Part model, mm, in its own coordinate system. A direction names the side the tool comes from. Give positions to 0.01 mm unless a question says otherwise; leave off trailing zeros. Loops run counter-clockwise (first coordinate to the right, second up) from the corner with the lowest first, then second, coordinate; pieces in that order, holes last. Notation, with made-up numbers: M 10,44 L 29,44 A21 cw 29,54 Z; hole C 77,81.5 d10. An arc over 180 degrees is marked long. Put each result on its own line as item: value. Start each with the question number.
```python
from build123d import *

# Parameters (mm, degrees)
SKETCH001_W      = 31
SKETCH001_H      = 36
EXTRUDE002_DEPTH = 16
SKETCH_W         = 33
SKETCH_H         = 38
EXTRUDE_DEPTH    = 18
FILLET_R         = 1
FILLET001_R      = 2
FILLET002_R      = 1


with BuildPart() as inside:
    # Sketch001 (on Face6 of Extrude) → Extrude002 (new body)
    with BuildSketch(Plane.XY.offset(18)):
        with Locations((16.5, 19)):
            Rectangle(SKETCH001_W, SKETCH001_H)
    extrude(amount=-EXTRUDE002_DEPTH)


with BuildPart() as body:
    # Sketch → Extrude (new body)
    with BuildSketch(Plane.XY):
        with Locations((16.5, 19)):
            Rectangle(SKETCH_W, SKETCH_H)
    extrude(amount=EXTRUDE_DEPTH)

    # Cut: cut Inside
    add(inside.part, mode=Mode.SUBTRACT)

    # Fillet
    fillet_edges = [body.edges().sort_by_distance(p)[0] for p in [
        (16.5, 37, 2),
        (32, 19, 2),
        (1, 19, 2),
        (16.5, 1, 2),
    ]]
    fillet(fillet_edges, radius=FILLET_R)

    # Fillet001
    fillet001_edges = [body.edges().sort_by_distance(p)[0] for p in [
        (0, 19, 0),
        (16.5, 0, 0),
        (16.5, 38, 0),
        (33, 19, 0),
    ]]
    fillet(fillet001_edges, radius=FILLET001_R)

    # Fillet002
    fillet002_edges = [body.edges().sort_by_distance(p)[0] for p in [
        (33, 38, 10),
        (33, 0, 10),
        (0, 0, 10),
        (0, 38, 10),
    ]]
    fillet(fillet002_edges, radius=FILLET002_R)


solid = body.part
```
1) Band-saw the part on A-A on x = 8. Give the cut face in (y, z), then the cut area to 3 significant figures.
2) Mould opens along X. For faces 1 (the flat face through (0, 19, 10)), 2 (the cylindrical face through (16.717, 36.715, 2.301)), 3 (the cylindrical face through (16.717, 1.285, 2.301)), 4 (the flat face through (16, 38, 10)) say: +X half, -X half, draft (parallel to the pull), parting line (faces both ways), or undercut.
3) Which spindle directions (+Z, -Z, +X, -X, +Y, -Y) get a long thin tool onto all of the face, cutting with end or side? Do faces 5 (the flat face through (16, 1, 11)), 6 (the cylindrical face through (0.285, 37.699, 10.112)). Say none if no direction does.
4) Pin check, flat tip, straight feed: pin 1 Ø6 at (x, y) = (27, 13.5) entering from +Z. Stop position of the tip, or through.
5) Band-saw the part on C-C on y = 30. Give the cut face in (x, z), then the cut area to 3 significant figures.
6) Wall check: L1, parallel to Y at x = 4, z = 15.5; L2, parallel to X at y = 12.5, z = 6; L3, parallel to Z at x = 13.5, y = 23. Give the ranges that are in metal, low to high.
7) Band-saw the part on B-B on z = 11.25. Give the cut face in (x, y), then the cut area to 3 significant figures.
Evaluation:
1. outline: M 0,2 A2 ccw 2,0 L 36,0 A2 ccw 38,2 L 38,18 L 37,18 L 37,3 A1 cw 36,2 L 2,2 A1 cw 1,3 L 1,18 L 0,18 Z
1. area: 107 mm2
2. face 1: -X half
2. face 2: undercut
2. face 3: undercut
2. face 4: draft
3. face 5: +Z
3. face 6: +Z, -Z, -X, +Y
4. pin 1: z = 2
5. outline: M 0,2 A2 ccw 2,0 L 31,0 A2 ccw 33,2 L 33,18 L 32,18 L 32,3 A1 cw 31,2 L 2,2 A1 cw 1,3 L 1,18 L 0,18 Z
5. area: 96.7 mm2
6. L1: 0 to 1, 37 to 38
6. L2: 0 to 1, 32 to 33
6. L3: 0 to 2
7. outline: M 0,1 A1 ccw 1,0 L 32,0 A1 ccw 33,1 L 33,37 A1 ccw 32,38 L 1,38 A1 ccw 0,37 Z; hole M 1,1 L 32,1 L 32,37 L 1,37 Z
7. area: 137 mm2
